Answer from the drawing. Dimensions are ordinates in mm from the lowest x, y and z of the part. Round coordinates to 2 decimals unless told otherwise and drop trailing zeros. Loops run counter-clockwise (first coordinate to the right, second up) from the corner with the lowest first, then second, coordinate; pieces in that order, holes last.
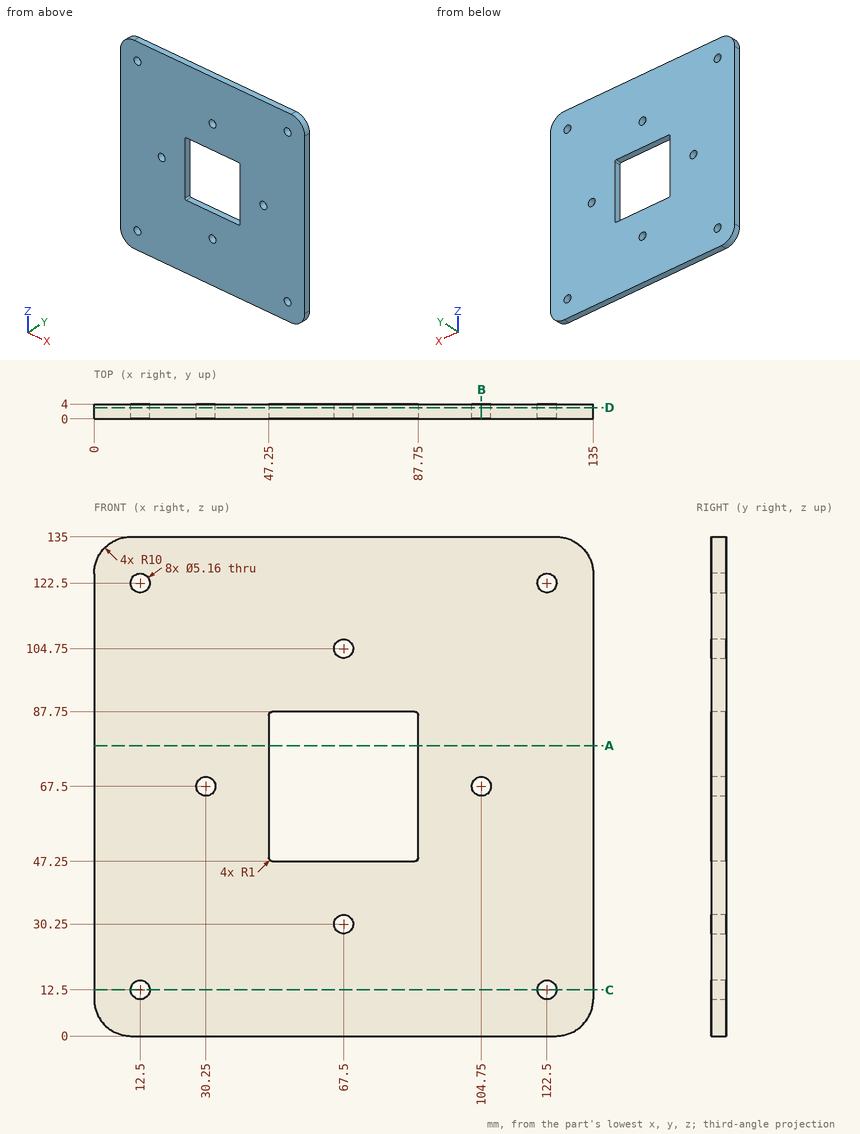
1. Consider probe 1 along X at (y, z) = (1.75, 122.5); probe 2 along Z at (x, y) = (49.5, 3.8). Determine where each line is inside the solid, lowest interval first.
Answer key:
probe 1: x = 0 to 9.92, 15.08 to 119.92, 125.08 to 135
probe 2: z = 0 to 47.25, 87.75 to 135
2. Find section C-C (z = 12.5). Write down the section's boundary in (x, y).
Answer key:
outline: (0, 0) - (9.92, 0) - (9.92, 4) - (0, 4) - close; (15.08, 0) - (119.92, 0) - (119.92, 4) - (15.08, 4) - close; (125.08, 0) - (135, 0) - (135, 4) - (125.08, 4) - close
3. Find section D-D (y = 3). Give the number of separate pieces and of enclosed holes in the cut face, then the cut area to 3 significant figures.
Answer key:
separate pieces: 1
enclosed holes: 9
area: 16,300 mm2
4. Find section B-B (x = 104.75). Write down the section's boundary in (y, z).
Answer key:
outline: (0, 0) - (4, 0) - (4, 64.92) - (0, 64.92) - close; (0, 70.08) - (4, 70.08) - (4, 135) - (0, 135) - close
5. Find section A-A (z = 78.5). Write down the section's boundary in (x, y), then the cut area to 3 significant figures.
Answer key:
outline: (0, 0) - (47.25, 0) - (47.25, 4) - (0, 4) - close; (87.75, 0) - (135, 0) - (135, 4) - (87.75, 4) - close
area: 378 mm2
